For this review, take the finished solid that the model builds, in its own axes (mm). A direction names the side the tool comes from. Coordinates: 2 decimals unless noted, no trailing zeros. Loops run counter-clockwise (first coordinate to the right, second up) from the corner with the lowest first, then second, coordinate; pieces in that order, holes last. Notation, with made-up numbers: M 89,16.25 L 109,16.25 A34 ccw 109,49.25 Z; hole C 44.5,-25 d3. An arc over 180 degrees is marked long. Answer as a JSON object with one key per item and string values. Group by question number.
Item 1: Insertion check: pin 1 (1.5 mm diameter, centred on x = 5, y = 25.5, fed in from +Z); pin 2 (8.5 mm diameter, centred on y = 15.875, z = 111.125, fed in from -X). Each pin has a flat end and moves straight along its axis. Give the tip position at first contact, or say it passes through.
Item 2: Mouldability with a two-part tool opening along Y and no side actions: class faces 3 (the face through (30.84, 30.8, 62.61)), 4 (the face through (16, 0, 63)), 5 (the face through (16, 2, 0)), 6 (the face through (30.14, 15.462, 114.273)) as +Y half, -Y half, draft (parallel to the pull), parting line (faces both ways), or undercut.
Item 3: Tool access review of faces 1 (the face through (28.575, 16, 63)), 2 (the face through (0, 16, 63)): name each direction out of +Z, -Z, +X, -X, +Y, -Y from which nothing blocks a thin tool from reaching the whole face with its end or side.
Item 4: Add section A-A (x = 24.5). State the section outline as (y, z) points (3 decimals), then the cut area to 3 significant figures.
Item 5: Wall thickness on L1, parallel to Y at x = 26.5, z = 76 (3 decimals); L2, parallel to X at y = 4, z = 48.5: over which ranges is each line inside the solid? List them lowest first. Write a range as from..to.
from build123d import *

# Parameters (mm, degrees)
F1_DEPTH = 127
F3_DEPTH = 127
F4_R     = 3.175
F4_R_2   = 2.994617
F5_DEPTH = 31.75


with BuildPart() as f1:
    # F0 (on Top) → F1 (new body)
    with BuildSketch(Plane.XY):
        with BuildLine():
            ThreePointArc((0, 3.175), (0.929936, 0.929936), (3.175, 0))
            Line((3.175, 0), (28.575, 0))
            ThreePointArc((28.575, 0), (30.820064, 0.929936), (31.75, 3.175))
            Line((31.75, 3.175), (31.75, 28.575))
            ThreePointArc((31.75, 28.575), (30.820064, 30.820064), (28.575, 31.75))
            Line((28.575, 31.75), (3.175, 31.75))
            ThreePointArc((3.175, 31.75), (0.929936, 30.820064), (0, 28.575))
            Line((0, 28.575), (0, 3.175))
        make_face()
    extrude(amount=F1_DEPTH)

    # F2 (on Top) → F3 (cut)
    with BuildSketch(Plane.XY):
        with BuildLine():
            ThreePointArc((3.175, 4.7625), (3.639968, 3.639968), (4.7625, 3.175))
            Line((4.7625, 3.175), (26.9875, 3.175))
            ThreePointArc((26.9875, 3.175), (28.110032, 3.639968), (28.575, 4.7625))
            Line((28.575, 4.7625), (28.575, 26.9875))
            ThreePointArc((28.575, 26.9875), (28.110032, 28.110032), (26.9875, 28.575))
            Line((26.9875, 28.575), (4.7625, 28.575))
            ThreePointArc((4.7625, 28.575), (3.639968, 28.110032), (3.175, 26.9875))
            Line((3.175, 26.9875), (3.175, 4.7625))
        make_face()
    extrude(amount=F3_DEPTH, mode=Mode.SUBTRACT)

    # F4 (on Right) → F5 (cut)
    with BuildSketch(Plane.YZ):
        with Locations((15.875, 111.125)):
            Circle(F4_R)
        with Locations((15.875, 98.425)):
            Circle(F4_R_2)
    extrude(amount=F5_DEPTH, mode=Mode.SUBTRACT)


solid = f1.part
From the geometry:
{
 "1": {"pin 1": "passes through", "pin 2": "stops at x = 0"},
 "2": {"face 3": "+Y half", "face 4": "-Y half", "face 5": "draft", "face 6": "undercut"},
 "3": {"face 1": "+Z, -Z", "face 2": "+Z, -Z, -X, +Y, -Y"},
 "4": {"outline": "M 0,0 L 3.175,0 L 3.175,127 L 0,127 Z; M 28.575,0 L 31.75,0 L 31.75,127 L 28.575,127 Z", "area": "806 mm²"},
 "5": {"L1": "y = 0..3.175, 28.575..31.75", "L2": "x = 0..3.37, 28.38..31.75"}
}
